Geometry check sheet. Reference: the model listing, model coordinates, mm. A direction names the side the tool comes from. Coordinates: 2 decimals unless noted, no trailing zeros. Write each loop counter-clockwise with the first axis right and the second up, starting at its lowest first coordinate (ties: lowest second). Pieces come first, ordered by that corner, then holes.
from build123d import *

# Parameters (mm, degrees)
SKETCH3_W           = 130
SKETCH3_H           = 10
BOSS_EXTRUDE1_DEPTH = 2
SKETCH4_R           = 1.5
BOSS_EXTRUDE2_DEPTH = 17


with BuildPart() as part:
    # Sketch3 → Boss-Extrude1 (new body)
    with BuildSketch(Plane(origin=(0, 0, 0), x_dir=(1, 0, 0), z_dir=(0, 1, 0))):
        Rectangle(SKETCH3_W, SKETCH3_H)
    extrude(amount=BOSS_EXTRUDE1_DEPTH)

    # Sketch4 → Boss-Extrude2 (add)
    with BuildSketch(Plane(origin=(0, 2, 0), x_dir=(1, 0, 0), z_dir=(0, 1, 0))):
        with Locations(Location((-60, 0, 0), (0, 0, 90))):
            Circle(SKETCH4_R)
    boss_extrude2 = extrude(amount=BOSS_EXTRUDE2_DEPTH)

    # Mirror1: Boss-Extrude2 across plane
    add(boss_extrude2.mirror(Plane.ZY))


solid = part.part
1. Draft check along X on faces 3 (the flat face through (65, 1, 0)), 4 (the flat face through (-1, 2, 0)), 5 (the flat face through (-1, 1, -5)). Enter one of: released by +X, released by -X, zero draft, split by the parting line, or undercut.
Computed values:
face 3: released by +X
face 4: undercut
face 5: zero draft
2. Access from +Z, -Z, +X, -X, +Y, -Y to the whole of each face (thin tool, end or side, straight path). Record for faces 1 (the flat face through (-60, 19, 0)), 2 (the cylindrical face through (-61.487, 10.381, 0.195)).
Computed values:
face 1: +Z, -Z, +X, -X, +Y
face 2: +Y
3. Thickness scan on line 1 along X through (y, z) = (5.25, 0); line 2 along Y through (x, z) = (-19.5, -2.75); line 3 along X through (y, z) = (2.5, 1.25). Record the ranges inside material, lowest first.
Computed values:
line 1: x = -61.5 to -58.5, 58.5 to 61.5
line 2: y = 0 to 2
line 3: x = -60.83 to -59.17, 59.17 to 60.83
4. Sectioned sample at A-A, the plane y = 7.75. Record the boundary of the cut face in (x, z).
Computed values:
outline: circle Ø3 at (-60, 0); circle Ø3 at (60, 0)
5. Gauge pin test, flat ends, axial feed: pin 1 Ø6 at (x, z) = (34.5, -3) entering from -Y; pin 2 Ø1 at (y, z) = (4, 4) entering from +X; pin 3 Ø2 at (y, z) = (16.5, -2) entering from +X; pin 4 Ø5 at (x, z) = (13, -2) entering from +Y. Record the tip position at first contact, or that the pin passes through.
Computed values:
pin 1: stops at y = 0
pin 2: passes through
pin 3: stops at x = 61.12
pin 4: stops at y = 2
6. Sectioned sample at D-D, the plane x = 48. Record the boundary of the cut face in (y, z).
Computed values:
outline: (0, -5) - (2, -5) - (2, 5) - (0, 5) - close
7. Sectioned sample at C-C, the plane z = 0. Record the boundary of the cut face in (x, y), and give its area (3 significant figures).
Computed values:
outline: (-65, 0) - (65, 0) - (65, 2) - (61.5, 2) - (61.5, 19) - (58.5, 19) - (58.5, 2) - (-58.5, 2) - (-58.5, 19) - (-61.5, 19) - (-61.5, 2) - (-65, 2) - close
area: 362 mm2
8. Sectioned sample at B-B, the plane x = -60. Record the boundary of the cut face in (y, z).
Computed values:
outline: (0, -5) - (2, -5) - (2, -1.5) - (19, -1.5) - (19, 1.5) - (2, 1.5) - (2, 5) - (0, 5) - close
